Build history of the part. All positions in model axes, mm. Give positions to 0.01 mm unless a question says otherwise; leave off trailing zeros. Loops run counter-clockwise (first coordinate to the right, second up) from the corner with the lowest first, then second, coordinate; pieces in that order, holes last. Notation, with made-up numbers: (16.5, 48.5) - (65.5, 48.5) arc R33 cw to (65.5, 82.5) - close; hole circle Ø1 at (-13, 61.5). An arc over 180 degrees is marked (long way). Return JSON: item names as keys, results as strings. Group by question number.
1) Drill centre lines: probe 1 along Y at (x, z) = (0, 2.95); probe 2 along X at (y, z) = (494, 2.6); probe 3 along Y at (x, z) = (0.75, 2.5). Where is each one in solid material? Low to high. Write a range as from..to.
2) Slice it at B-B (y = 145.5). List the corners of the cut face in (x, z), and give its area (3 significant figures).
3) Drop flat-ended pins along their axis: pin 1 (2.5 mm diameter, centred on x = 0, y = 494, fed in from -Z); pin 2 (3 mm diameter, centred on y = 103.5, z = -2, fed in from +X); pin 3 (3 mm diameter, centred on x = 0, z = 0, fed in from +Y) (3 decimals); pin 4 (4 mm diameter, centred on y = 269.5, z = 3, fed in from -X). Give the stop position or say it passes through.
4) Slice it at A-A (z = 0). List the corners of the cut face in (x, y).
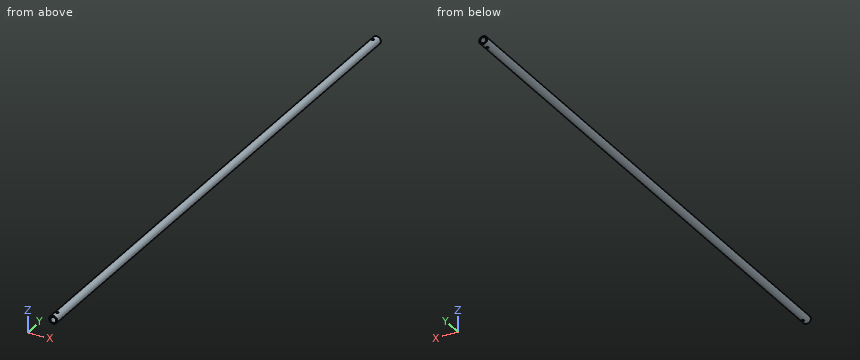
Autodesk Inventor part; units mm, degrees
ref_plane "YZ Plane" through (0, 0, 0) normal (1, 0, 0) x (0, 1, 0)
ref_plane "XZ Plane" through (0, 0, 0) normal (0, 1, 0) x (-1, 0, 0)
ref_plane "XY Plane" through (0, 0, 0) normal (0, 0, 1) x (1, 0, 0)
sketch "Sketch2" plane through (0, 0, 0) normal (0, 1, 0) x (-1, 0, 0)
  circle A0 centre (0, 0) radius 3.5
  circle A1 centre (0, 0) radius 2.5
  dimension "d91" = 7
  dimension "d92" = 5
extrude "Extrusion5" add sketch "Sketch2" along normal blind 500
sketch "Sketch3" plane through (0, 0, 0) normal (0, 0, 1) x (1, 0, 0)
  line L0 (0, 0) -> (0, 6) construction
  circle A0 centre (0, 6) radius 1
  line L1 (3.5, 500) -> (-3.5, 500)
  line L2 (0, 500) -> (0, 494)
  circle A1 centre (0, 494) radius 1
  dimension "d95" = 6
  dimension "d96" = 2
  dimension "d97" = 6
  dimension "d98" = 2
extrude "Extrusion6" cut sketch "Sketch3" along normal blind 10 and the other way blind 10
properties part number "airfoil"
Results:
{
 "1": {"probe 1": "0..5, 7..493, 495..500", "probe 2": "-2.34..-1, 1..2.34", "probe 3": "0..5.34, 6.66..493.34, 494.66..500"},
 "2": {"outline": "circle Ø7 at (0, 0); hole circle Ø5 at (0, 0)", "area": "18.8 mm2"},
 "3": {"pin 1": "z = -3.5", "pin 2": "x = 3.46", "pin 3": "through", "pin 4": "x = -3.35"},
 "4": {"outline": "(-3.5, 0) - (-2.5, 0) - (-2.5, 500) - (-3.5, 500) - close; (2.5, 0) - (3.5, 0) - (3.5, 500) - (2.5, 500) - close"}
}
